The model under review builds one solid part; all positions refer to its coordinate system, in mm. Face numbers are marked on the shaded views. A direction names the side the tool comes from. Round coordinates to 2 decimals unless told otherwise and drop trailing zeros. Write each loop counter-clockwise with the first axis right and the second up, starting at its lowest first coordinate (ties: lowest second). Pieces come first, ordered by that corner, then holes. Notation, with made-up numbers: (-11.5, 45) -> (45.5, 45) arc R6 cw to (45.5, 54) -> close; hole circle Ø5 at (69.5, 59.5). An arc over 180 degrees is marked (long way). Return JSON: item names as keys, results as strings. Group by question number.
1. Mouldability with a two-part tool opening along X and no side actions: class the marked faces 3, 4 and 5 as pulls with the +X half, pulls with the -X half, needs draft (parallel to the pull), parting line crosses it, or undercut.
2. Tool access review of the marked faces 1 and 2: name each direction out of +Z, -Z, +X, -X, +Y, -Y from which nothing blocks a thin tool from reaching the whole face with its end or side.
3. Take a section at D-D, the plane y = 18.5. Write out the cut boundary in (x, z), then the cut area to 3 significant figures.
4. Take a section at C-C, the plane z = 14.5. Write out the cut boundary in (x, y), then the cut area to 3 significant figures.
5. Take a section at A-A, the plane x = 0. Write out the cut boundary in (y, z) (3 decimals), then the cut area to 3 significant figures.
6. For line 1 along Y through (x, z) = (0, 6.25); line 2 along Y through (x, z) = (0, 2.5); line 3 along Z through (x, y) = (-6.5, -8.5), list the stretches that pass through material, from the lowest coordinate up. Write a range as from..to.
7. Clearance check with flat-ended pins moving along their axes: P1, Ø19, axis at x = 0, y = -3, coming from the -Z side; P2, Ø1.5, axis at y = -9.5, z = 13, coming from the -X side; P3, Ø1, axis at x = -1.5, z = 34.5, coming from the +Y side; P4, Ø5, axis at y = -6.5, z = 8.5, coming from the -X side. State where each tip first meets the part, or that it passes through.
from build123d import *

# Parameters (mm, degrees)
SKETCH1_R           = 24.6126
BOSS_EXTRUDE1_DEPTH = 4.826
SKETCH2_R           = 9.9187
BOSS_EXTRUDE2_DEPTH = 45.2374
SKETCH3_R           = 8.7122
CUT_EXTRUDE1_DEPTH  = 9.525


with BuildPart() as part:
    # Sketch1 → Boss-Extrude1 (new body)
    with BuildSketch(Plane.XY):
        Circle(SKETCH1_R)
    extrude(amount=BOSS_EXTRUDE1_DEPTH)

    # Sketch2 → Boss-Extrude2 (add)
    with BuildSketch(Plane.XY):
        Circle(SKETCH2_R)
    extrude(amount=BOSS_EXTRUDE2_DEPTH)

    # Sketch3 → Cut-Extrude1 (cut)
    with BuildSketch(Plane.XY):
        Circle(SKETCH3_R)
    extrude(amount=CUT_EXTRUDE1_DEPTH, mode=Mode.SUBTRACT)


solid = part.part
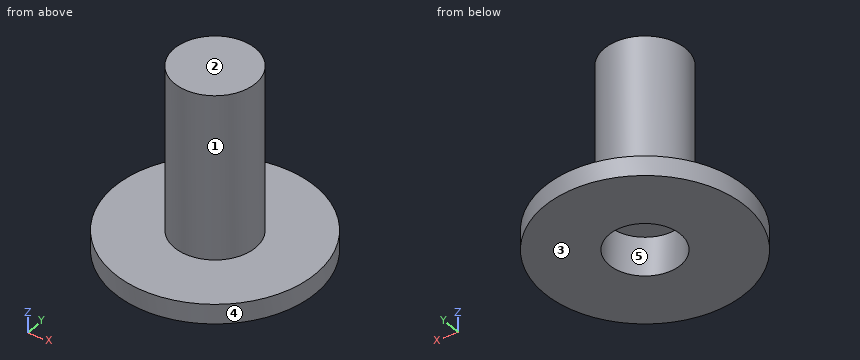
Output:
{
 "1": {"face 3": "needs draft", "face 4": "parting line crosses it", "face 5": "undercut"},
 "2": {"face 1": "+Z", "face 2": "+Z, +X, -X, +Y, -Y"},
 "3": {"outline": "(-16.23, 0) -> (16.23, 0) -> (16.23, 4.83) -> (-16.23, 4.83) -> close", "area": "157 mm^2"},
 "4": {"outline": "circle Ø19.84 at (0, 0)", "area": "309 mm^2"},
 "5": {"outline": "(-24.613, 0) -> (-8.712, 0) -> (-8.712, 9.525) -> (8.712, 9.525) -> (8.712, 0) -> (24.613, 0) -> (24.613, 4.826) -> (9.919, 4.826) -> (9.919, 45.237) -> (-9.919, 45.237) -> (-9.919, 4.826) -> (-24.613, 4.826) -> close", "area": "873 mm^2"},
 "6": {"line 1": "y = -9.92..-8.71, 8.71..9.92", "line 2": "y = -24.61..-8.71, 8.71..24.61", "line 3": "z = 0..4.83"},
 "7": {"P1": "stops at z = 0", "P2": "stops at x = -4.67", "P3": "stops at y = 9.87", "P4": "stops at x = -9.08"}
}
